Design review of the part built by this model. Coordinates are the model's own, in mm. A direction names the side the tool comes from. Round coordinates to 2 decimals unless told otherwise and drop trailing zeros. Order: outer loops, then holes, each group sorted by start corner. A loop starts at its lowest first (then second) coordinate and runs counter-clockwise, first axis right, second up. Notation, with made-up numbers: (87, 68) - (122, 68) arc R23 ccw to (122, 90) - close; hole circle Ø5 at (11.5, -14.75). An arc over 180 degrees is marked (long way). Answer as a JSON object with one key per item and string values. Group by question number.
from build123d import *

# Parameters (mm, degrees)
F0_W      = 104.8863008618
F0_H      = 51.5389591455
F1_DEPTH  = 25.4
F2_R      = 5.08
F3_W      = 79.4863008618
F3_H      = 15.1469794668
F4_DEPTH  = 19.05
F6_DEPTH  = 25.4
F7_W      = 6.35
F7_H      = 51.5389591455
F8_DEPTH  = 19.05
F9_W      = 22.86
F9_H      = 25.7694795728
F10_DEPTH = 19.05
F11_R     = 5.08


with BuildPart() as f1:
    # F0 (on Top) → F1 (new body)
    with BuildSketch(Plane.XY):
        Rectangle(F0_W, F0_H)
    extrude(amount=F1_DEPTH)

    # F2
    f2_edges = [f1.edges().sort_by_distance(p)[0] for p in [
        (-52.44315, 25.76948, 12.7),
        (52.44315, 25.76948, 12.7),
    ]]
    fillet(f2_edges, radius=F2_R)

    # F3 (on face) → F4 (cut)
    with BuildSketch(Plane.XY.offset(25.4)):
        with Locations((0, -18.1959898394)):
            Rectangle(F3_W, F3_H)
    extrude(amount=-F4_DEPTH, mode=Mode.SUBTRACT)

    # F5 (on face) → F6 (cut)
    with BuildSketch(Plane.XY.offset(25.4)):
        with BuildLine():
            ThreePointArc((-18.1976626917, 25.7694795728), (0, 7.571816881), (18.1976626917, 25.7694795728))
            Line((18.1976626917, 25.7694795728), (-18.1976626917, 25.7694795728))
        make_face()
    extrude(amount=-F6_DEPTH, mode=Mode.SUBTRACT)

    # F7 (on face) → F8 (cut)
    with BuildSketch(Plane.XY.offset(25.4)):
        with Locations((-49.2681504309, 0)):
            Rectangle(F7_W, F7_H)
        with Locations((49.2681504309, 0)):
            Rectangle(F7_W, F7_H)
    extrude(amount=-F8_DEPTH, mode=Mode.SUBTRACT)

    # F9 (on face) → F10 (cut)
    with BuildSketch(Plane.XY.offset(25.4)):
        with Locations((-34.6631504309, 12.8847397864)):
            Rectangle(F9_W, F9_H)
        with Locations((34.6631504309, 12.8847397864)):
            Rectangle(F9_W, F9_H)
    extrude(amount=-F10_DEPTH, mode=Mode.SUBTRACT)

    # F11
    f11_edges = [f1.edges().sort_by_distance(p)[0] for p in [
        (-23.23315, 0, 15.875),
        (23.23315, 0, 15.875),
    ]]
    fillet(f11_edges, radius=F11_R)


solid = f1.part
1. Take a section at A-A, the plane y = -2.5. Give the boundary of the cut face in (x, z).
2. Take a section at B-B, the plane z = 4.25. Give the boundary of the cut face in (x, y).
3. Take a section at D-D, the plane y = -18. Give the boundary of the cut face in (x, z), then the cut area to 3 significant figures.
4. Tool access review of faces 4 (the cylindrical face through (-24.68, 1.53, 15.74)), 5 (the flat face through (46.093, -13, 16)), 6 (the cylindrical face through (50.995, 24.242, 3.219)), 7 (the flat face through (23.233, 15, 16)): name each direction out of +Z, -Z, +X, -X, +Y, -Y from which nothing blocks a thin tool from reaching the whole face with its end or side.
5. To check wall thickness, follow line 1 (X direction, y = -15, z = 10); line 2 (Z direction, x = 24.5, y = -17); line 3 (Y direction, x = -21, z = 6.75). State the ranges of each line that lie inside material, in increasing order. Write a range as from..to.
6. Take a section at C-C, the plane x = 0. Give the boundary of the cut face in (y, z).
7. Clearance check with flat-ended pins moving along their axes: P1, Ø10, axis at x = -33, y = -18.5, coming from the +Z side; P2, Ø12, axis at y = -20.5, z = 11.5, coming from the -X side; P3, Ø3, axis at x = 1.5, z = 18.5, coming from the -Y side; P4, Ø5.5, axis at y = 19, z = 18, coming from the -X side. State where each tip first meets the part, or that it passes through.
8. Mouldability with a two-part tool opening along X and no side actions: class faces 1 (the flat face through (-46.093, -13, 16)), 2 (the flat face through (-39.743, -18, 16)), 3 (the flat face through (-41, 6, 6.35)) as pulls with the +X half, pulls with the -X half, needs draft (parallel to the pull), parting line crosses it, or undercut.
Response values:
{
 "1": {"outline": "(-52.44, 0) - (52.44, 0) - (52.44, 6.35) - (46.09, 6.35) - (46.09, 25.4) - (-46.09, 25.4) - (-46.09, 6.35) - (-52.44, 6.35) - close"},
 "2": {"outline": "(-52.44, -25.77) - (52.44, -25.77) - (52.44, 20.69) arc R5.08 ccw to (47.36, 25.77) - (18.2, 25.77) arc R18.2 cw to (-18.2, 25.77) - (-47.36, 25.77) arc R5.08 ccw to (-52.44, 20.69) - close"},
 "3": {"outline": "(-52.44, 0) - (52.44, 0) - (52.44, 6.35) - (46.09, 6.35) - (46.09, 25.4) - (39.74, 25.4) - (39.74, 6.35) - (-39.74, 6.35) - (-39.74, 25.4) - (-46.09, 25.4) - (-46.09, 6.35) - (-52.44, 6.35) - close", "area": "908 mm2"},
 "4": {"face 4": "+Z, -X, +Y", "face 5": "+Z, +X, +Y, -Y", "face 6": "+Z, -Z, +X, +Y", "face 7": "+Z, +X, +Y"},
 "5": {"line 1": "-46.09..-39.74, 39.74..46.09", "line 2": "0..6.35", "line 3": "-10.62..25.77"},
 "6": {"outline": "(-25.77, 0) - (7.57, 0) - (7.57, 25.4) - (-10.62, 25.4) - (-10.62, 6.35) - (-25.77, 6.35) - close"},
 "7": {"P1": "z = 6.35", "P2": "x = -52.44", "P3": "y = -10.62", "P4": "x = -23.23"},
 "8": {"face 1": "pulls with the -X half", "face 2": "undercut", "face 3": "needs draft"}
}
